Geometry check sheet. Reference: the model listing, model coordinates, mm. Face numbers are marked on the shaded views. A direction names the side the tool comes from. Give positions to 0.01 mm unless a question says otherwise; leave off trailing zeros. Write each loop counter-clockwise with the first axis right and the second up, starting at its lowest first coordinate (ties: lowest second). Pieces come first, ordered by that corner, then holes. Notation, with made-up numbers: (49.5, 15.5) -> (56.5, 15.5) arc R28 cw to (56.5, 54.5) -> close; hole circle Ø11 at (28.25, -14.5). An arc over 180 degrees is marked (long way). Write item = value, one per line. Start each with the question number.
1. Depth check by flat-ended pin: P1, Ø5, axis at x = -43, z = -8.5, coming from the +Y side; P2, Ø3.5, axis at x = 41.5, y = -1, coming from the -Z side; P3, Ø4, axis at y = 4, z = -3, coming from the +X side. Enter the tip coordinate at first touch or a pass-through.
2. Set-up check for the marked faces 3, 4, 5 and 6: record each of +Z, -Z, +X, -X, +Y, -Y from which the full face is reachable in a straight line by a thin tool's end or side.
3. Cross-section at C-C, the plane x = 15. Record the cut outline in (y, z), plus the area to 3 significant figures.
4. Thickness scan on line 1 along Z through (x, y) = (41, -0.75); line 2 along Z through (x, y) = (32, 2.5); line 3 along X through (y, z) = (-1.5, 0.5). Record the ranges inside material, lowest first.
5. Cross-section at B-B, the plane z = -20. Record the cut outline in (x, y).
6. Cross-section at D-D, the plane y = 4. Record the cut outline in (x, z).
7. Mould release check, pull along X, two halves, no side actions. Record for the marked faces 1 and 2: pulls with the +X half, pulls with the -X half, needs draft (parallel to the pull), parting line crosses it, or undercut.
8. Cross-section at A-A, the plane x = -41. Record the cut outline in (y, z), plus the area to 3 significant figures.
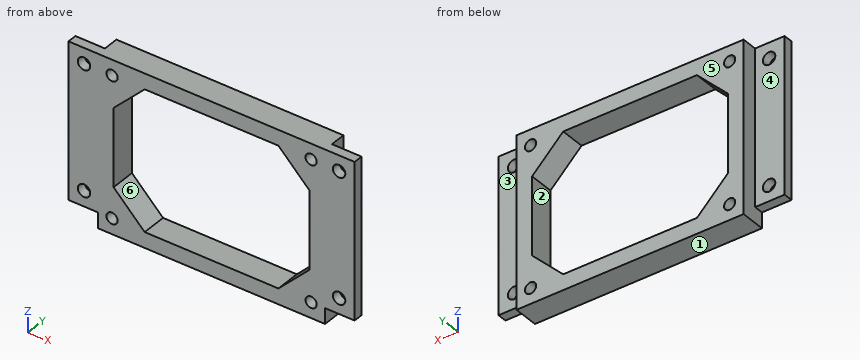
```python
from build123d import *

# Parameters (mm, degrees)
SKETCH1_W                = 73
SKETCH1_H                = 50
BOSS_EXTRUDE1_DEPTH      = 5
SKETCH2_W                = 92
SKETCH2_H                = 50
BOSS_EXTRUDE2_DEPTH      = 3
M3_CLEARANCE_HOLE1_D     = 4
M3_CLEARANCE_HOLE1_DEPTH = 10
M3_CLEARANCE_HOLE1_TIP   = 1.201721238
SKETCH9_W                = 73
SKETCH9_H                = 8
BOSS_EXTRUDE3_DEPTH      = 5
M3_CLEARANCE_HOLE3_D     = 3.6
M3_CLEARANCE_HOLE3_DEPTH = 10
M3_CLEARANCE_HOLE3_TIP   = 1.081549114
CUT_EXTRUDE1_DEPTH       = 9


with BuildPart() as part:
    # Sketch1 → Boss-Extrude1 (new body)
    with BuildSketch(Plane(origin=(0, 0, 0), x_dir=(1, 0, 0), z_dir=(0, 1, 0))):
        Rectangle(SKETCH1_W, SKETCH1_H)
    extrude(amount=BOSS_EXTRUDE1_DEPTH)

    # Sketch2 → Boss-Extrude2 (add)
    with BuildSketch(Plane.XZ):
        Rectangle(SKETCH2_W, SKETCH2_H)
    extrude(amount=BOSS_EXTRUDE2_DEPTH)

    # M3 Clearance Hole1
    with Locations(Plane(origin=(0, 0, 0), x_dir=(1, 0, 0), z_dir=(0, 1, 0))):
        with Locations((-41, 20), (-41, -20), (41, 20), (41, -20)):
            Hole(M3_CLEARANCE_HOLE1_D / 2, depth=M3_CLEARANCE_HOLE1_DEPTH)
            with Locations((0, 0, -(M3_CLEARANCE_HOLE1_DEPTH + M3_CLEARANCE_HOLE1_TIP / 2))):  # 118° drill point
                Cone(0, M3_CLEARANCE_HOLE1_D / 2, M3_CLEARANCE_HOLE1_TIP, mode=Mode.SUBTRACT)

    # Sketch9 → Boss-Extrude3 (add)
    with BuildSketch(Plane(origin=(0, 0, -25), x_dir=(-1, 0, 0), z_dir=(0, 0, -1))):
        with Locations((0, 1)):
            Rectangle(SKETCH9_W, SKETCH9_H)
    extrude(amount=BOSS_EXTRUDE3_DEPTH)

    # M3 Clearance Hole3
    with Locations(Plane(origin=(0, 5, 0), x_dir=(1, 0, 0), z_dir=(0, 1, 0))):
        with Locations((32, -20), (-32, 25), (32, 25), (-32, -20)):
            Hole(M3_CLEARANCE_HOLE3_D / 2, depth=M3_CLEARANCE_HOLE3_DEPTH)
            with Locations((0, 0, -(M3_CLEARANCE_HOLE3_DEPTH + M3_CLEARANCE_HOLE3_TIP / 2))):  # 118° drill point
                Cone(0, M3_CLEARANCE_HOLE3_D / 2, M3_CLEARANCE_HOLE3_TIP, mode=Mode.SUBTRACT)

    # Sketch12 → Cut-Extrude1 (cut, through all)
    with BuildSketch(Plane(origin=(0, 5, 0), x_dir=(1, 0, 0), z_dir=(0, 1, 0))):
        Polygon((21.5, -20), (31.5, -10), (31.5, 15), (21.5, 25), (-21.5, 25), (-31.5, 15), (-31.5, -10), (-21.5, -20), align=None)
    extrude(amount=-CUT_EXTRUDE1_DEPTH, mode=Mode.SUBTRACT)


solid = part.part
```
Answers:
q1.P1 = 0
q1.P2 = -25
q1.P3 = 36.5
q2.face_3 = +Z, -Z, +X, +Y
q2.face_4 = +Z, -Z, -X, +Y
q2.face_5 = +Z, -Z, +X, -X, +Y
q2.face_6 = +Y, -Y
q3.outline = (-3, -30) -> (5, -30) -> (5, -25) -> (-3, -25) -> close; (-3, 20) -> (5, 20) -> (5, 25) -> (-3, 25) -> close
q3.area = 80.0 mm^2
q4.line_1 = -25 to -22, -18 to 18, 22 to 25
q4.line_2 = -30 to -26.8, -23.2 to 18.2, 21.8 to 25
q4.line_3 = -46 to -31.5, 31.5 to 46
q5.outline = (-46, -3) -> (-43, -3) -> (-43, 0) -> (-46, 0) -> close; (-39, -3) -> (-26.5, -3) -> (-26.5, 5) -> (-36.5, 5) -> (-36.5, 0) -> (-39, 0) -> close; (26.5, -3) -> (39, -3) -> (39, 0) -> (36.5, 0) -> (36.5, 5) -> (26.5, 5) -> close; (43, -3) -> (46, -3) -> (46, 0) -> (43, 0) -> close
q6.outline = (-36.5, -30) -> (36.5, -30) -> (36.5, 25) -> (-36.5, 25) -> close; hole circle Ø3.6 at (-32, -25); hole circle Ø3.6 at (-32, 20); hole (-31.5, -15) -> (-21.5, -25) -> (21.5, -25) -> (31.5, -15) -> (31.5, 10) -> (21.5, 20) -> (-21.5, 20) -> (-31.5, 10) -> close; hole circle Ø3.6 at (32, -25); hole circle Ø3.6 at (32, 20)
q7.face_1 = needs draft
q7.face_2 = undercut
q8.outline = (-3, -25) -> (0, -25) -> (0, -22) -> (-3, -22) -> close; (-3, -18) -> (0, -18) -> (0, 18) -> (-3, 18) -> close; (-3, 22) -> (0, 22) -> (0, 25) -> (-3, 25) -> close
q8.area = 126 mm^2
